Could you check a few things on this model? Use its own coordinates, in mm. A direction names the side the tool comes from. Coordinates: 2 decimals unless noted, no trailing zeros. Write each loop counter-clockwise with the first axis right and the second up, starting at its lowest first coordinate (ties: lowest second). Pieces come first, ordered by that corner, then holes.
```python
from build123d import *

# Parameters (mm, degrees)
BOSS_EXTRUDE3_DEPTH             = 10
BOSS_EXTRUDE5_DEPTH             = 105
FILLET2_R                       = 9
BOSS_EXTRUDE7_DEPTH             = 25.7
FILLET3_R                       = 10
FILLET4_R                       = 10
CUT_EXTRUDE4_DEPTH              = 1.5
FILLET5_R                       = 3
CUT_EXTRUDE5_DEPTH              = 20
FILLET6_R                       = 10
CUT_EXTRUDE6_REACH              = 188.714
SKETCH13_R                      = 5
M4X0_7_TAPPED_HOLE2_D           = 3.3
M4X0_7_TAPPED_HOLE2_DEPTH       = 5
SM1_TAPPED_HOLE1_D              = 25.4
SM1_TAPPED_HOLE1_DEPTH          = 5
M4X0_7_TAPPED_HOLE1_D           = 3.3
M4X0_7_TAPPED_HOLE1_DEPTH       = 8
M4X0_7_TAPPED_HOLE1_TIP         = 0.991420021
M2X0_4_TAPPED_HOLE1_D           = 1.6
M2X0_4_TAPPED_HOLE1_DEPTH       = 5.2
M2X0_4_TAPPED_HOLE1_TIP         = 0.480688495
M3X0_5_TAPPED_HOLE1_D           = 2.5
M3X0_5_TAPPED_HOLE1_DEPTH       = 7.5
M3X0_5_TAPPED_HOLE1_TIP         = 0.751075774
F_3_0MM_DOWEL_HOLE1_D           = 3
F_3_0MM_DOWEL_HOLE1_DEPTH       = 5.2
F_3_0MM_DOWEL_HOLE1_TIP         = 0.901290929
M3X0_5_TAPPED_HOLE2_D           = 2.5
M3X0_5_TAPPED_HOLE2_DEPTH       = 5
M3X0_5_TAPPED_HOLE3_D           = 2.5
M3X0_5_TAPPED_HOLE3_DEPTH       = 7.5
M3X0_5_TAPPED_HOLE3_TIP         = 0.751075774
F_1_16_0_0625_DOWEL_HOLE1_D     = 1.5875
F_1_16_0_0625_DOWEL_HOLE1_DEPTH = 5.2
F_1_16_0_0625_DOWEL_HOLE1_TIP   = 0.476933116
F_3_0MM_DOWEL_HOLE2_D           = 3
F_3_0MM_DOWEL_HOLE2_DEPTH       = 5.2
F_3_0MM_DOWEL_HOLE2_TIP         = 0.901290929
M3X0_5_TAPPED_HOLE4_D           = 2.5
M3X0_5_TAPPED_HOLE4_DEPTH       = 7.5
M3X0_5_TAPPED_HOLE4_TIP         = 0.751075774
CUT_EXTRUDE7_DEPTH              = 103.5
M5X0_8_TAPPED_HOLE2_D           = 4.2
M5X0_8_TAPPED_HOLE2_DEPTH       = 5
M5X0_8_TAPPED_HOLE3_D           = 4.2
M5X0_8_TAPPED_HOLE3_DEPTH       = 5


with BuildPart() as part:
    # Sketch1 → Boss-Extrude3 (new body)
    with BuildSketch(Plane(origin=(0, 0, 0), x_dir=(1, 0, 0), z_dir=(0, 1, 0))):
        Polygon((-99.454594588, 85.287259619), (-99.454594588, 27.580704883), (24.630684429, -93.704474274), (87.259436127, -29.629818302), (87.259436127, 85.287259619), align=None)
    extrude(amount=BOSS_EXTRUDE3_DEPTH)

    # Sketch6 → Boss-Extrude5 (add)
    with BuildSketch(Plane(origin=(0, 10, 0), x_dir=(1, 0, 0), z_dir=(0, 1, 0))):
        Polygon((-99.454594588, 85.287259619), (-99.454594588, 27.580704883), (24.630684429, -93.704474274), (87.259436127, -29.629818302), (87.259436127, 85.287259619), align=None)
        Polygon((82.259436127, 80.287259619), (-94.454594588, 80.287259619), (-94.454594588, 29.68527495), (24.549996611, -86.63386684), (82.259436127, -27.592094762), align=None, mode=Mode.SUBTRACT)
    extrude(amount=BOSS_EXTRUDE5_DEPTH)

    # Fillet2
    fillet2_edges = [part.edges().sort_by_distance(p)[0] for p in [
        (82.259436127, 62.5, -80.287259619),
        (-94.454594588, 62.5, -80.287259619),
        (-94.454594588, 62.5, -29.68527495),
        (24.549996611, 62.5, 86.63386684),
        (82.259436127, 62.5, 27.592094762),
    ]]
    fillet(fillet2_edges, radius=FILLET2_R)

    # Sketch9 → Boss-Extrude7 (add)
    with BuildSketch(Plane(origin=(0, 10, 0), x_dir=(1, 0, 0), z_dir=(0, 1, 0))):
        Polygon((-9.164109107, 80.287259619), (-9.164109107, 16.274353327), (-44.132452564, -19.501301083), (-96.380135247, 31.56736399), (-96.380135247, 80.287259619), align=None)
    extrude(amount=BOSS_EXTRUDE7_DEPTH)

    # Fillet3
    fillet3_edges = [part.edges().sort_by_distance(p)[0] for p in [
        (-44.132452564, 22.85, 19.501301083),
    ]]
    fillet(fillet3_edges, radius=FILLET3_R)

    # Fillet4
    fillet4_edges = [part.edges().sort_by_distance(p)[0] for p in [
        (-9.164109107, 22.85, -80.287259619),
    ]]
    fillet(fillet4_edges, radius=FILLET4_R)

    # Sketch10 → Cut-Extrude4 (cut)
    with BuildSketch(Plane(origin=(0, 115, 0), x_dir=(1, 0, 0), z_dir=(0, 1, 0))):
        Polygon((-97.954594588, 28.212075903), (24.606478083, -91.583292044), (85.759436127, -29.01850124), (85.759436127, 83.787259619), (-97.954594588, 83.787259619), align=None)
    extrude(amount=-CUT_EXTRUDE4_DEPTH, mode=Mode.SUBTRACT)

    # Fillet5
    fillet5_edges = [part.edges().sort_by_distance(p)[0] for p in [
        (-97.954594588, 114.25, -28.212075903),
        (-97.954594588, 114.25, -83.787259619),
        (85.759436127, 114.25, -83.787259619),
        (85.759436127, 114.25, 29.01850124),
        (24.606478083, 114.25, 91.583292044),
    ]]
    fillet(fillet5_edges, radius=FILLET5_R)

    # Sketch12 → Cut-Extrude5 (cut)
    with BuildSketch(Plane.XZ):
        Polygon((-86.029052321, -30.238498612), (-44.83183875, 10.029061474), (-15.886944756, -19.584080646), (-15.886944756, -74.947835353), (-86.029052321, -74.947835353), align=None)
    extrude(amount=-CUT_EXTRUDE5_DEPTH, mode=Mode.SUBTRACT)

    # Fillet6
    fillet6_edges = [part.edges().sort_by_distance(p)[0] for p in [
        (-86.029052321, 10, -74.947835353),
        (-86.029052321, 10, -30.238498612),
        (-44.83183875, 10, 10.029061474),
        (-15.886944756, 10, -19.584080646),
        (-15.886944756, 10, -74.947835353),
    ]]
    fillet(fillet6_edges, radius=FILLET6_R)

    # Sketch13 → Cut-Extrude6 (cut, up to next)
    with BuildSketch(Plane(origin=(87.259436127, 0, 0), x_dir=(0, 0, -1), z_dir=(1, 0, 0)), mode=Mode.PRIVATE) as cut_extrude6_sk1:
        with Locations((2.612649558, 61.1)):
            Circle(SKETCH13_R)
    cut_extrude6_tool1 = extrude(cut_extrude6_sk1.sketch, amount=-CUT_EXTRUDE6_REACH, mode=Mode.PRIVATE) & part.part
    add(cut_extrude6_tool1.solids().sort_by_distance((87.259436, 61.1, -2.61265))[0], mode=Mode.SUBTRACT)

    # M4x0.7 Tapped Hole2
    with Locations(Plane(origin=(59.436420011, 0, 58.095181851), x_dir=(0.698991962, 0, -0.715129525), z_dir=(0.715129525, 0, 0.698991962))):
        with Locations((2.431115729, 37.767314098), (2.431115729, 84.532685902), (-24.568884271, 84.532685902), (-24.568884271, 37.767314098)):
            Hole(M4X0_7_TAPPED_HOLE2_D / 2, depth=M4X0_7_TAPPED_HOLE2_DEPTH)

    # SM1 Tapped Hole1
    with Locations(Plane(origin=(59.436420011, 0, 58.095181851), x_dir=(0.698991962, 0, -0.715129525), z_dir=(0.715129525, 0, 0.698991962))):
        with Locations((-10.825880291, 61.15)):
            Hole(SM1_TAPPED_HOLE1_D / 2, depth=SM1_TAPPED_HOLE1_DEPTH)

    # M4x0.7 Tapped Hole1
    with Locations(Plane(origin=(0, 35.7, 0), x_dir=(1, 0, 0), z_dir=(0, 1, 0))):
        with Locations((-76.250393956, 74.820995384), (-89.615612831, 42.554502711)):
            Hole(M4X0_7_TAPPED_HOLE1_D / 2, depth=M4X0_7_TAPPED_HOLE1_DEPTH)
            with Locations((0, 0, -(M4X0_7_TAPPED_HOLE1_DEPTH + M4X0_7_TAPPED_HOLE1_TIP / 2))):  # 118° drill point
                Cone(0, M4X0_7_TAPPED_HOLE1_D / 2, M4X0_7_TAPPED_HOLE1_TIP, mode=Mode.SUBTRACT)

    # M2x0.4 Tapped Hole1
    with Locations(Plane(origin=(0, 10, 0), x_dir=(1, 0, 0), z_dir=(0, 1, 0))):
        with Locations((5.789584185, 54.312649558), (25.789584185, 54.312649558), (5.789584185, 34.312649558), (25.789584185, 34.312649558)):
            Hole(M2X0_4_TAPPED_HOLE1_D / 2, depth=M2X0_4_TAPPED_HOLE1_DEPTH)
            with Locations((0, 0, -(M2X0_4_TAPPED_HOLE1_DEPTH + M2X0_4_TAPPED_HOLE1_TIP / 2))):  # 118° drill point
                Cone(0, M2X0_4_TAPPED_HOLE1_D / 2, M2X0_4_TAPPED_HOLE1_TIP, mode=Mode.SUBTRACT)

    # M3x0.5 Tapped Hole1
    with Locations(Plane(origin=(0, 10, 0), x_dir=(1, 0, 0), z_dir=(0, 1, 0))):
        with Locations((53.486513194, 36.740704463), (53.486513194, 17.338730644)):
            Hole(M3X0_5_TAPPED_HOLE1_D / 2, depth=M3X0_5_TAPPED_HOLE1_DEPTH)
            with Locations((0, 0, -(M3X0_5_TAPPED_HOLE1_DEPTH + M3X0_5_TAPPED_HOLE1_TIP / 2))):  # 118° drill point
                Cone(0, M3X0_5_TAPPED_HOLE1_D / 2, M3X0_5_TAPPED_HOLE1_TIP, mode=Mode.SUBTRACT)

    # Ø3.0mm Dowel Hole1
    with Locations(Plane(origin=(0, 10, 0), x_dir=(1, 0, 0), z_dir=(0, 1, 0))):
        with Locations((73.986513194, 2.338730644), (53.486513194, 53.338730644)):
            Hole(F_3_0MM_DOWEL_HOLE1_D / 2, depth=F_3_0MM_DOWEL_HOLE1_DEPTH)
            with Locations((0, 0, -(F_3_0MM_DOWEL_HOLE1_DEPTH + F_3_0MM_DOWEL_HOLE1_TIP / 2))):  # 118° drill point
                Cone(0, F_3_0MM_DOWEL_HOLE1_D / 2, F_3_0MM_DOWEL_HOLE1_TIP, mode=Mode.SUBTRACT)

    # M3x0.5 Tapped Hole2
    with Locations(Plane(origin=(87.259436127, 0, 0), x_dir=(0, 0, -1), z_dir=(1, 0, 0))):
        with Locations((17.112649558, 75.6), (17.112649558, 46.6), (-11.887350442, 46.6), (-11.887350442, 75.6)):
            Hole(M3X0_5_TAPPED_HOLE2_D / 2, depth=M3X0_5_TAPPED_HOLE2_DEPTH)

    # M3x0.5 Tapped Hole3
    with Locations(Plane(origin=(0, 35.7, 0), x_dir=(1, 0, 0), z_dir=(0, 1, 0))):
        with Locations((-19.601854144, 60.718472071), (-19.601854144, 33.456137846)):
            Hole(M3X0_5_TAPPED_HOLE3_D / 2, depth=M3X0_5_TAPPED_HOLE3_DEPTH)
            with Locations((0, 0, -(M3X0_5_TAPPED_HOLE3_DEPTH + M3X0_5_TAPPED_HOLE3_TIP / 2))):  # 118° drill point
                Cone(0, M3X0_5_TAPPED_HOLE3_D / 2, M3X0_5_TAPPED_HOLE3_TIP, mode=Mode.SUBTRACT)

    # 1/16 (0.0625) Dowel Hole1
    with Locations(Plane(origin=(0, 35.7, 0), x_dir=(1, 0, 0), z_dir=(0, 1, 0))):
        with Locations((-81.65008966, 47.846563072), (-74.359970274, 65.446468166)):
            Hole(F_1_16_0_0625_DOWEL_HOLE1_D / 2, depth=F_1_16_0_0625_DOWEL_HOLE1_DEPTH)
            with Locations((0, 0, -(F_1_16_0_0625_DOWEL_HOLE1_DEPTH + F_1_16_0_0625_DOWEL_HOLE1_TIP / 2))):  # 118° drill point
                Cone(0, F_1_16_0_0625_DOWEL_HOLE1_D / 2, F_1_16_0_0625_DOWEL_HOLE1_TIP, mode=Mode.SUBTRACT)

    # Ø3.0mm Dowel Hole2
    with Locations(Plane(origin=(0, 35.7, 0), x_dir=(1, 0, 0), z_dir=(0, 1, 0))):
        with Locations((-19.575203756, 47.747012064), (-31.16172375, 14.167066106)):
            Hole(F_3_0MM_DOWEL_HOLE2_D / 2, depth=F_3_0MM_DOWEL_HOLE2_DEPTH)
            with Locations((0, 0, -(F_3_0MM_DOWEL_HOLE2_DEPTH + F_3_0MM_DOWEL_HOLE2_TIP / 2))):  # 118° drill point
                Cone(0, F_3_0MM_DOWEL_HOLE2_D / 2, F_3_0MM_DOWEL_HOLE2_TIP, mode=Mode.SUBTRACT)

    # M3x0.5 Tapped Hole4
    with Locations(Plane(origin=(0, 113.5, 0), x_dir=(1, 0, 0), z_dir=(0, 1, 0))):
        with Locations((-94.273905994, 79.93319266), (82.766021198, 80.287259619), (24.2404501, -86.105034639)):
            Hole(M3X0_5_TAPPED_HOLE4_D / 2, depth=M3X0_5_TAPPED_HOLE4_DEPTH)
            with Locations((0, 0, -(M3X0_5_TAPPED_HOLE4_DEPTH + M3X0_5_TAPPED_HOLE4_TIP / 2))):  # 118° drill point
                Cone(0, M3X0_5_TAPPED_HOLE4_D / 2, M3X0_5_TAPPED_HOLE4_TIP, mode=Mode.SUBTRACT)

    # Sketch44 → Cut-Extrude7 (cut)
    with BuildSketch(Plane(origin=(0, 113.5, 0), x_dir=(1, 0, 0), z_dir=(0, 1, 0))):
        with BuildLine():
            Line((10.581140502, 83.777152415), (35.2341862, 83.777152415))
            ThreePointArc((35.2341862, 83.777152415), (45.2341862, 73.777152415), (35.2341862, 63.777152415))
            Line((35.2341862, 63.777152415), (10.581140502, 63.777152415))
            ThreePointArc((10.581140502, 63.777152415), (0.581140502, 73.777152415), (10.581140502, 83.777152415))
        make_face()
    extrude(amount=-CUT_EXTRUDE7_DEPTH, mode=Mode.SUBTRACT)

    # M5x0.8 Tapped Hole2
    with Locations(Plane(origin=(59.436420011, 0, 58.095181851), x_dir=(0.698991962, 0, -0.715129525), z_dir=(0.715129525, 0, 0.698991962))):
        with Locations((-10.825880291, 91.15), (-10.825880291, 31.15), (19.174119709, 61.15)):
            Hole(M5X0_8_TAPPED_HOLE2_D / 2, depth=M5X0_8_TAPPED_HOLE2_DEPTH)

    # M5x0.8 Tapped Hole3
    with Locations(Plane(origin=(59.436420011, 0, 58.095181851), x_dir=(0.698991962, 0, -0.715129525), z_dir=(0.715129525, 0, 0.698991962))):
        with Locations((-33.825880291, 95.15), (12.174119709, 95.15), (12.174119709, 27.15), (-33.825880291, 27.15)):
            Hole(M5X0_8_TAPPED_HOLE3_D / 2, depth=M5X0_8_TAPPED_HOLE3_DEPTH)


solid = part.part
```
Item 1: If we mould it in two halves opening along Y, with no side actions, what happens to faces 4 (the flat face through (87.259, 57, -27)), 5 (the flat face through (13, 0, -17)), 6 (the cylindrical face through (67.215, 28.569, 46.51))? For each: released by +Y, released by -Y, zero draft, split by the parting line, or undercut.
Item 2: Which directions (+Z, -Z, +X, -X, +Y, -Y) give clear straight access to the entire face, cutting with the end or side of a thin tool? Please do faces 1 (the cylindrical face through (84.79, 56.22, -1.53)), 2 (the cylindrical face through (-83.02, 10.14, -72.1)), 3 (the flat face through (58, 61, -80.287)).
Item 3: Will these pins go through, and if not, where does the flat tip stop? pin 1 Ø1.5 at (y, z) = (75.6, 11.89) entering from +X; pin 2 Ø4 at (x, z) = (53.49, -36.74) entering from +Y; pin 3 Ø2 at (x, z) = (-19.6, -33.46) entering from -Y.
Item 4: If I drill on line 1 along X through (y, z) = (23, -69.5); line 2 along X through (y, z) = (62.5, -57.5); line 3 along Z through (x, y) = (46, 52), over which ranges is the centre line in solid material (lowest first)?
Item 5: I want a section at B-B, the plane x = -48. List the corners of the cut face in (y, z) for me.
Item 6: I want a section at A-A, the plane y = 13. Count the separate pieces of the cut face and the enclosed holes in it, then the cut area to 3 significant figures.
Taken from the geometry:
1. face 4: zero draft
1. face 5: released by -Y
1. face 6: undercut
2. face 1: +X
2. face 2: -Y
2. face 3: +Y
3. pin 1: stops at x = -51.15
3. pin 2: stops at y = 10
3. pin 3: stops at y = 20
4. line 1: x = -99.45 to -9.16, 82.26 to 87.26
4. line 2: x = -99.45 to -94.45, 82.26 to 87.26
4. line 3: z = -85.29 to -80.29
5. outline: (0, -85.29) - (115, -85.29) - (115, -83.79) - (113.5, -83.79) - (113.5, -80.29) - (35.7, -80.29) - (35.7, 15.72) - (113.5, 15.72) - (113.5, 20.62) - (115, 20.62) - (115, 22.71) - (0, 22.71) - (0, 5.43) - (20, 5.43) - (20, -74.95) - (0, -74.95) - close
6. separate pieces: 1
6. enclosed holes: 2
6. area: 4,990 mm2
